from build123d import *

# Parameters (mm, degrees)
F0_R     = 4.7625
F1_DEPTH = 38.1
F2_DEPTH = 25.4


with BuildPart() as f1:
    # F0 (on Right) → F1 (new body)
    with BuildSketch(Plane.YZ):
        with BuildLine():
            Line((0, 12.7), (-127, 12.7))
            Line((-127, 12.7), (-127, -12.7))
            Line((-127, -12.7), (0, -12.7))
            Line((0, -12.7), (0, -4.7625))
            ThreePointArc((0, -4.7625), (-4.7625, 0), (0, 4.7625))
            Line((0, 4.7625), (0, 12.7))
        make_face()
        with Locations((-114.3, 0)):
            Circle(F0_R, mode=Mode.SUBTRACT)
        with BuildLine():
            Line((177.8, 12.7), (0, 12.7))
            Line((0, 12.7), (0, 4.7625))
            ThreePointArc((0, 4.7625), (3.3675960454, 3.3675960454), (4.7625, 0))
            ThreePointArc((4.7625, 0), (3.3675960454, -3.3675960454), (0, -4.7625))
            Line((0, -4.7625), (0, -12.7))
            Line((0, -12.7), (177.8, -12.7))
            Line((177.8, -12.7), (177.8, 12.7))
        make_face()
        with Locations((165.1, 0)):
            Circle(F0_R, mode=Mode.SUBTRACT)
    extrude(amount=F1_DEPTH)

    # F0 (on Right) → F2 (join)
    with BuildSketch(Plane.YZ):
        with BuildLine():
            Line((0, 12.7), (-127, 12.7))
            Line((-127, 12.7), (-127, -12.7))
            Line((-127, -12.7), (0, -12.7))
            Line((0, -12.7), (0, -4.7625))
            ThreePointArc((0, -4.7625), (-4.7625, 0), (0, 4.7625))
            Line((0, 4.7625), (0, 12.7))
        make_face()
        with Locations((-114.3, 0)):
            Circle(F0_R, mode=Mode.SUBTRACT)
        with BuildLine():
            Line((177.8, 12.7), (0, 12.7))
            Line((0, 12.7), (0, 4.7625))
            ThreePointArc((0, 4.7625), (3.3675960454, 3.3675960454), (4.7625, 0))
            ThreePointArc((4.7625, 0), (3.3675960454, -3.3675960454), (0, -4.7625))
            Line((0, -4.7625), (0, -12.7))
            Line((0, -12.7), (177.8, -12.7))
            Line((177.8, -12.7), (177.8, 12.7))
        make_face()
        with Locations((165.1, 0)):
            Circle(F0_R, mode=Mode.SUBTRACT)
    extrude(amount=F2_DEPTH)


solid = f1.part
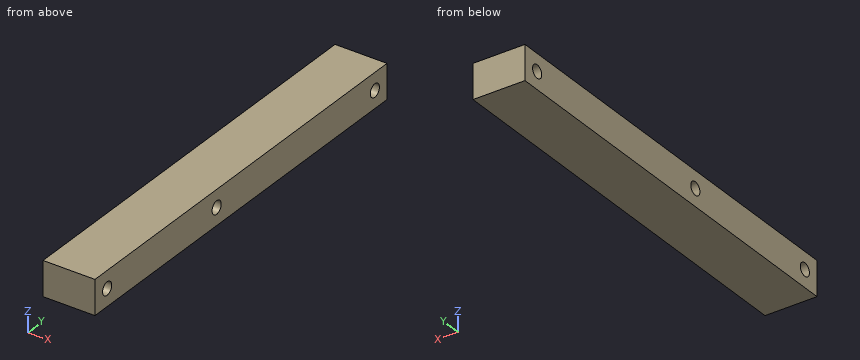
Can you work these out from the model? Positions are in its coordinate system, mm. Coordinates: 2 decimals unless noted, no trailing zeros. Order: outer loops, then holes, each group sorted by start corner. A loop starts at its lowest first (then second) coordinate and runs counter-clockwise, first axis right, second up. Notation, with made-up numbers: (72, 33.5) - (112, 33.5) arc R16 ccw to (112, 45.5) - close; hole circle Ø7 at (15.5, 62.25). An arc over 180 degrees is marked (long way). Answer as a JSON object with one key per item and string values. Group by question number.
Q1. Will this pin go through, and if not, where does the flat tip stop? P1, Ø5.5, axis at y = -114.3, z = 0, coming from the -X side.
Q2. Imagine slicing it at C-C (z = 0). Please give me the cut outline in (x, y), and give its area (3 significant figures).
Q3. I need wall thicknesses on line 1 (Y direction, x = 9, z = 0.75); line 2 (Z direction, x = 10, y = -114.3); line 3 (Y direction, x = 10, z = 3). Which ranges of each line are inside material? Lowest first, please. Write a range as from..to.
Q4. Imagine slicing it at B-B (y = -114.3). Please give me the cut outline in (x, z).
Q5. Imagine slicing it at A-A (x = 30). Please give me the cut outline in (y, z) (1 decimal).
Determined:
{
 "1": {"P1": "passes through"},
 "2": {"outline": "(0, -127) - (38.1, -127) - (38.1, -119.06) - (0, -119.06) - close; (0, -109.54) - (38.1, -109.54) - (38.1, -4.76) - (0, -4.76) - close; (0, 4.76) - (38.1, 4.76) - (38.1, 160.34) - (0, 160.34) - close; (0, 169.86) - (38.1, 169.86) - (38.1, 177.8) - (0, 177.8) - close", "area": "10,500 mm2"},
 "3": {"line 1": "y = -127..-119, -109.6..-4.7, 4.7..160.4, 169.8..177.8", "line 2": "z = -12.7..-4.76, 4.76..12.7", "line 3": "y = -127..-118, -110.6..-3.7, 3.7..161.4, 168.8..177.8"},
 "4": {"outline": "(0, -12.7) - (38.1, -12.7) - (38.1, -4.76) - (0, -4.76) - close; (0, 4.76) - (38.1, 4.76) - (38.1, 12.7) - (0, 12.7) - close"},
 "5": {"outline": "(-127, -12.7) - (177.8, -12.7) - (177.8, 12.7) - (-127, 12.7) - close; hole circle Ø9.5 at (-114.3, 0); hole circle Ø9.5 at (0, 0); hole circle Ø9.5 at (165.1, 0)"}
}
